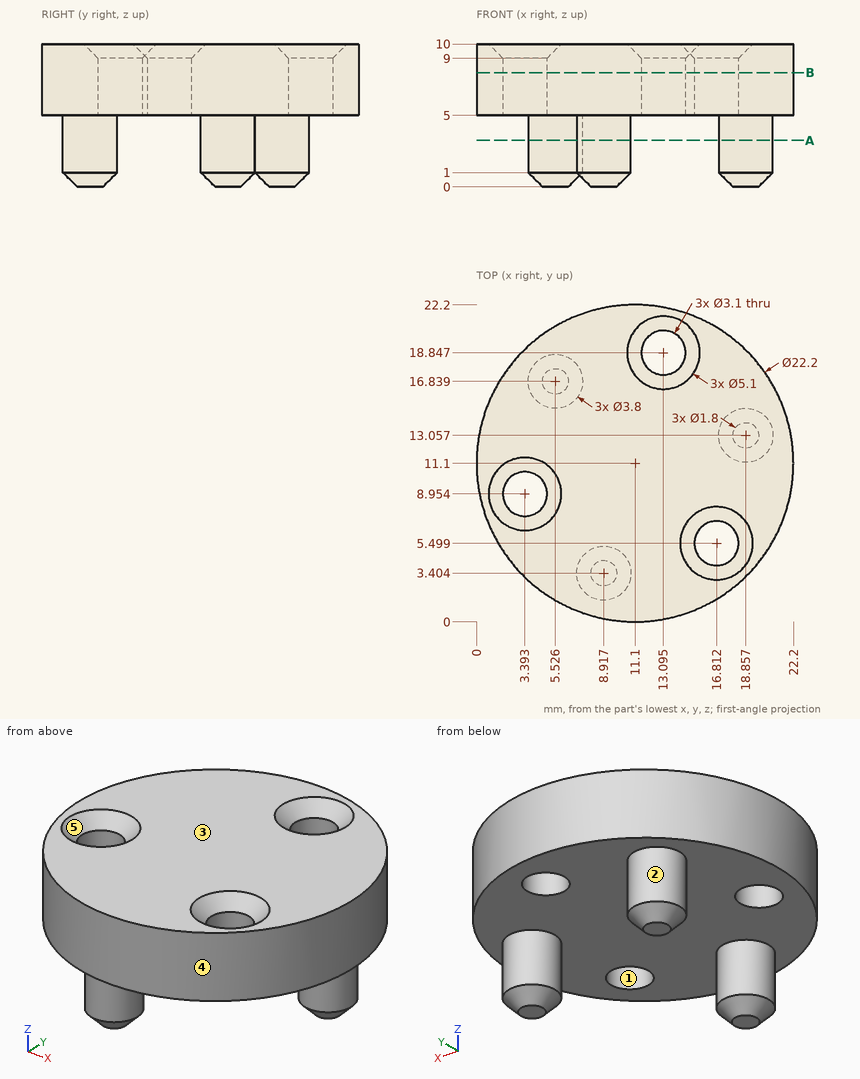
The drawing under review shows one solid part. Ordinate dimensions are in mm from its lowest x, y, z. A direction names the side the tool comes from. Give positions to 0.01 mm unless a question says otherwise; leave off trailing zeros. Loops run counter-clockwise (first coordinate to the right, second up) from the corner with the lowest first, then second, coordinate; pieces in that order, holes last. Notation, with made-up numbers: M 24,25.5 L 68,25.5 A37 ccw 68,61.5 Z; hole C 16,64 d2. An arc over 180 degrees is marked long. One line per item, written item: value. Start each with the question number.
Q1. Machinability: for the marked faces 1 and 2, which of the approach directions +Z, -Z, +X, -X, +Y, -Y give a long, thin tool a straight path to every point of the face, cutting with its end or side? Answer none if there is none.
Q2. Add section B-B (z = 8). Count the separate pieces of the cut face and the enclosed holes in it.
Q3. For L1, parallel to Z at x = 12.25, y = 5.5; L2, parallel to Y at x = 4.75, z = 8.5 (1 decimal); L3, parallel to Y at x = 7.25, z = 3.5 (1 decimal), list the stretches that pass through material, from the lowest coordinate up.
Q4. Clearance check with flat-ended pins moving along their axes: pin 1 Ø4 at (y, z) = (4.5, 4.5) entering from -X; pin 2 Ø5 at (x, y) = (3.39, 8.95) entering from -Z; pin 3 Ø1 at (y, z) = (16.5, 2.5) entering from +X. State where each tip first meets the part, or that it passes through.
Q5. Add section A-A (z = 3.25). Give the boundary of the cut face in (x, y).
Q6. Draft analysis for pull direction Y (two halves, no side actions). For the marked faces 3, 4 and 5, state which applies: released by +Y, released by -Y, zero draft, split by the parting line, or undercut.
Reply:
1. face 1: +Z, -Z
1. face 2: -Z
2. separate pieces: 1
2. enclosed holes: 3
3. L1: 5 to 10
3. L2: 2 to 8.2, 9.7 to 20.2
3. L3: 2.5 to 4.3, 16 to 17.6
4. pin 1: x = 1.03
4. pin 2: z = 5
4. pin 3: x = 7.43
5. outline: C 5.53,16.84 d3.8; C 8.92,3.4 d3.8; C 18.86,13.06 d3.8
6. face 3: zero draft
6. face 4: split by the parting line
6. face 5: undercut
